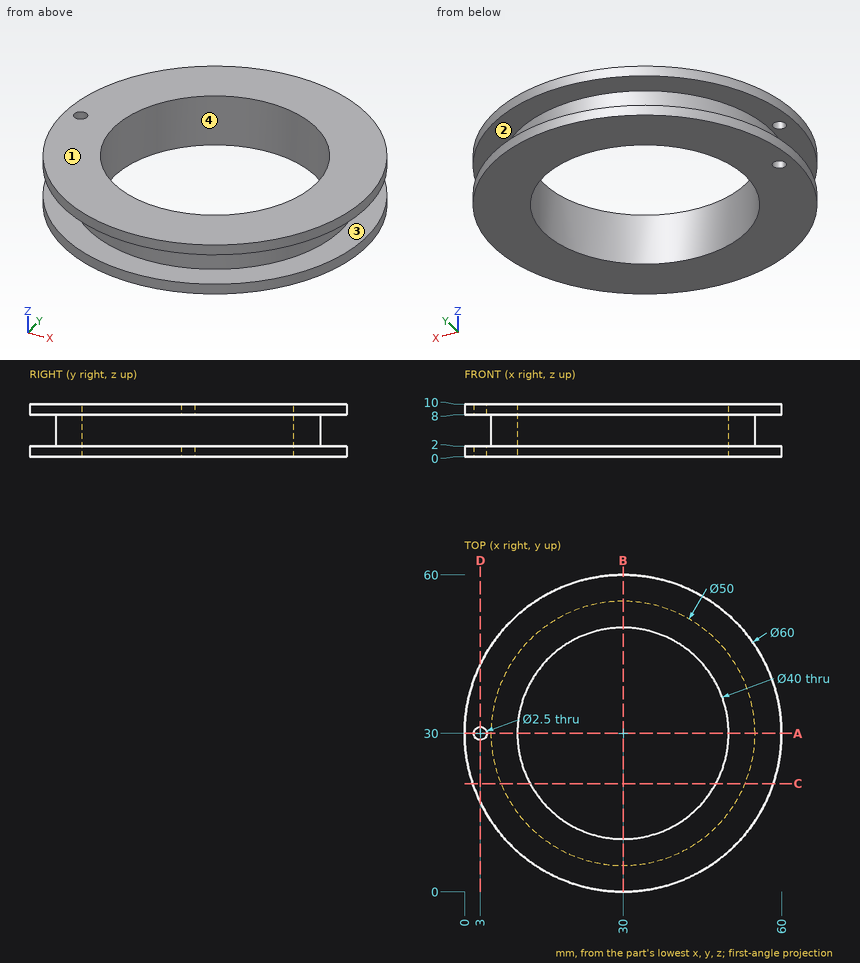
Design review of the part shown in the three views and the two pictorial views. Dimensions are in mm from the part's minimum x, y and z. A direction names the side the tool comes from. Give positions to 0.01 mm unless a question says otherwise; leave off trailing zeros. Write each loop counter-clockwise with the first axis right and the second up, starting at its lowest first coordinate (ties: lowest second). Pieces come first, ordered by that corner, then holes.
Item 1: Machinability: for the marked faces 1 and 2, which of the approach directions +Z, -Z, +X, -X, +Y, -Y give a long, thin tool a straight path to every point of the face, cutting with its end or side? Answer none if there is none.
Item 2: The part is to be moulded in two halves that separate along Y. For the marked faces 3 and 4, say which applies: +Y half, -Y half, draft (parallel to the pull), parting line (faces both ways), or undercut.
Item 3: Take a section at A-A (y = 30). Give the boundary of the cut face in (x, z), and give its area (3 significant figures).
Item 4: Take a section at D-D (x = 3). Give the boundary of the cut face in (y, z).
Item 5: Take a section at B-B (x = 30). Give the boundary of the cut face in (y, z).
Item 6: Wall thickness on probe 1 along Z at (x, y) = (54, 45.5); probe 2 along Y at (x, z) = (30, 5.75); probe 3 along Y at (x, z) = (3, 8.45): over which ranges is each line inside the solid? List them lowest first.
Item 7: Insertion check: P1, Ø6, axis at x = 7, z = 1, coming from the -Y side; P2, Ø6, axis at y = 30, z = 6.5, coming from the -X side; P3, Ø18, axis at x = 28.5, y = 33, coming from the -Z side; P4, Ø4, axis at x = 10.5, z = 1.5, coming from the -Y side. Each pin has a flat end and moves straight along its axis. Give the tip position at first contact, or say it passes through.
Item 8: Take a section at C-C (y = 20.5). Give the boundary of the cut face in (x, z), and give its area (3 significant figures).
Established:
1. face 1: +Z, +X, -X, +Y, -Y
1. face 2: none
2. face 3: draft
2. face 4: undercut
3. outline: (0, 0) - (1.75, 0) - (1.75, 2) - (0, 2) - close; (0, 8) - (1.75, 8) - (1.75, 10) - (0, 10) - close; (4.25, 0) - (10, 0) - (10, 10) - (4.25, 10) - (4.25, 8) - (5, 8) - (5, 2) - (4.25, 2) - close; (50, 0) - (60, 0) - (60, 2) - (55, 2) - (55, 8) - (60, 8) - (60, 10) - (50, 10) - close
3. area: 130 mm2
4. outline: (16.92, 0) - (28.75, 0) - (28.75, 2) - (16.92, 2) - close; (16.92, 8) - (28.75, 8) - (28.75, 10) - (16.92, 10) - close; (31.25, 0) - (43.08, 0) - (43.08, 2) - (31.25, 2) - close; (31.25, 8) - (43.08, 8) - (43.08, 10) - (31.25, 10) - close
5. outline: (0, 0) - (10, 0) - (10, 10) - (0, 10) - (0, 8) - (5, 8) - (5, 2) - (0, 2) - close; (50, 0) - (60, 0) - (60, 2) - (55, 2) - (55, 8) - (60, 8) - (60, 10) - (50, 10) - close
6. probe 1: z = 0 to 2, 8 to 10
6. probe 2: y = 5 to 10, 50 to 55
6. probe 3: y = 16.92 to 28.75, 31.25 to 43.08
7. P1: stops at y = 7.64
7. P2: stops at x = 0
7. P3: passes through
7. P4: stops at y = 5.63
8. outline: (1.54, 0) - (12.4, 0) - (12.4, 10) - (1.54, 10) - (1.54, 8) - (6.88, 8) - (6.88, 2) - (1.54, 2) - close; (47.6, 0) - (58.46, 0) - (58.46, 2) - (53.12, 2) - (53.12, 8) - (58.46, 8) - (58.46, 10) - (47.6, 10) - close
8. area: 153 mm2
